The listing builds one solid part. Answer for the finished solid, in the listing's coordinates (mm). Coordinates: 2 decimals unless noted, no trailing zeros. Order: outer loops, then holes, each group sorted by start corner. A loop starts at its lowest first (then second) coordinate and runs counter-clockwise, first axis right, second up. Notation, with made-up numbers: (0, -3) -> (40, -3) arc R19 ccw to (40, 13) -> close; hole circle Ø7 at (76.5, -28). An arc over 180 degrees is marked (long way). Write each question's results on one line, items separated by ' | '. Start each with the question number.
(1) The part is cut by section B-B, the plane z = 7.25. Give the vertices of the cut face in (x, y).
(2) The part is cut by section C-C, the plane y = 2.5. Give the vertices of the cut face in (x, z).
(3) Given pin 1 (2.5 mm diameter, centred on y = 3.5, z = 8, fed in from -X); pin 2 (0.8 mm diameter, centred on x = 1, z = 9.5, fed in from +Y); pin 3 (1.5 mm diameter, centred on y = 1.5, z = 5.5, fed in from -X), each flat-ended and moving along its own axis, determine where each tip first touches the part or whether it passes through.
(4) Straight lines are drawn through the part: L1, parallel to X at y = 1.85, z = 11; L2, parallel to Y at x = 1.4, z = 14.75; L3, parallel to Z at x = -0.1, y = 2.45. For each, find the intervals that lie inside material, in ascending order.
(5) The part is cut by section A-A, the plane y = 1.2. Give the vertices of the cut face in (x, z).
(6) The part is cut by section D-D, the plane z = 16. Give the vertices of the cut face in (x, y), then the cut area to 3 significant figures.
```python
from build123d import *

# Parameters (mm, degrees)
SKETCH2_W           = 18.2
SKETCH2_H           = 5
BOSS_EXTRUDE1_DEPTH = 1.5
SKETCH4_W           = 3.6
SKETCH4_H           = 0.6
CUT_EXTRUDE1_DEPTH  = 0.6
SKETCH5_W           = 3.3
SKETCH5_H           = 0.5
BOSS_EXTRUDE2_DEPTH = 0.2
BOSS_EXTRUDE5_DEPTH = 3.3
SKETCH9_R           = 0.06
CUT_EXTRUDE5_DEPTH  = 12
FILLET1_R           = 0.25


with BuildPart() as part:
    # Sketch2 → Boss-Extrude1 (new body)
    with BuildSketch(Plane(origin=(0, 0, 0), x_dir=(0, 0, -1), z_dir=(1, 0, 0))):
        with Locations((-9.1, 2.5)):
            Rectangle(SKETCH2_W, SKETCH2_H)
    extrude(amount=BOSS_EXTRUDE1_DEPTH)

    # Sketch3 → Revolve1 (revolve)
    with BuildSketch(Plane.XY.offset(11)):
        Polygon((0, 2.5), (0, 3.1), (-0.3, 3.1), (-0.3, 2.8), (-0.6, 2.8), (-0.6, 2.5), align=None)
    revolve(axis=Axis((0, 2.5, 11), (-1, 0, 0)))

    # Sketch4 → Cut-Extrude1 (cut)
    with BuildSketch(Plane.ZY):
        with Locations((7.7, 2.5)):
            Rectangle(SKETCH4_W, SKETCH4_H)
    extrude(amount=-CUT_EXTRUDE1_DEPTH, mode=Mode.SUBTRACT)

    # Sketch5 → Boss-Extrude2 (add)
    with BuildSketch(Plane.ZY):
        with Locations((9.35, 4.85)):
            Rectangle(SKETCH5_W, SKETCH5_H)
    boss_extrude2 = extrude(amount=BOSS_EXTRUDE2_DEPTH)

    # Sketch6 → Boss-Extrude5 (add)
    with BuildSketch(Plane.XY.offset(11)):
        with BuildLine():
            Line((-0.2, 5.1), (0, 5.1))
            ThreePointArc((0, 5.1), (-0.1, 5.2), (-0.2, 5.1))
        make_face()
    boss_extrude5 = extrude(amount=-BOSS_EXTRUDE5_DEPTH)

    # Sketch9 → Cut-Extrude5 (cut, through all)
    with BuildSketch(Plane.XY.offset(11)):
        with Locations((-0.1, 5.1)):
            Circle(SKETCH9_R)
    cut_extrude5 = extrude(amount=-CUT_EXTRUDE5_DEPTH, mode=Mode.SUBTRACT)

    # Mirror8: Boss-Extrude2, Boss-Extrude5, Cut-Extrude5 across plane
    add(boss_extrude2.mirror(Plane.ZX.offset(2.5)))
    add(boss_extrude5.mirror(Plane.ZX.offset(2.5)))
    add(cut_extrude5.mirror(Plane.ZX.offset(2.5)), mode=Mode.SUBTRACT)

    # Fillet1
    fillet1_edges = [part.edges().sort_by_distance(p)[0] for p in [
        (1.5, 2.5, 18.2),
        (0, 2.5, 18.2),
        (0, 2.5, 0),
        (1.5, 2.5, 0),
    ]]
    fillet(fillet1_edges, radius=FILLET1_R)


solid = part.part
```
Established:
1) outline: (0, 0) -> (1.5, 0) -> (1.5, 5) -> (0, 5) -> (0, 2.8) -> (0.6, 2.8) -> (0.6, 2.2) -> (0, 2.2) -> close
2) outline: (-0.6, 10.7) -> (-0.3, 10.7) -> (-0.3, 10.4) -> (0, 10.4) -> (0, 9.5) -> (0.6, 9.5) -> (0.6, 5.9) -> (0, 5.9) -> (0, 0.25) arc R0.25 ccw to (0.25, 0) -> (1.25, 0) arc R0.25 ccw to (1.5, 0.25) -> (1.5, 17.95) arc R0.25 ccw to (1.25, 18.2) -> (0.25, 18.2) arc R0.25 ccw to (0, 17.95) -> (0, 11.6) -> (-0.3, 11.6) -> (-0.3, 11.3) -> (-0.6, 11.3) -> close
3) pin 1: stops at x = -0.2 | pin 2: stops at y = 5 | pin 3: stops at x = 0
4) L1: x = 0 to 1.5 | L2: y = 0 to 5 | L3: z = 10.4 to 11.6
5) outline: (0, 0.25) arc R0.25 ccw to (0.25, 0) -> (1.25, 0) arc R0.25 ccw to (1.5, 0.25) -> (1.5, 17.95) arc R0.25 ccw to (1.25, 18.2) -> (0.25, 18.2) arc R0.25 ccw to (0, 17.95) -> close
6) outline: (0, 0) -> (1.5, 0) -> (1.5, 5) -> (0, 5) -> close | area: 7.50 mm^2
